```python
from build123d import *

# Parameters (mm, degrees)
BOSS_EXTRUDE1_DEPTH = 15
FILLET1_R           = 2.5


with BuildPart() as part:
    # Sketch1 → Boss-Extrude1 (new body)
    with BuildSketch(Plane.XY):
        with BuildLine():
            Line((4.569752453, 56.5222889), (27.069752453, 56.5222889))
            Line((27.069752453, 56.5222889), (27.069752453, 51.5222889))
            Line((27.069752453, 51.5222889), (4.569751288, 51.5222889))
            ThreePointArc((4.569751288, 51.5222889), (-15.430247547, 31.522287735), (4.569753619, 11.5222889))
            ThreePointArc((4.569753619, 11.5222889), (29.569753619, -13.4777111), (4.569753619, -38.4777111))
            Line((4.569753619, -38.4777111), (-17.930246381, -38.4777111))
            Line((-17.930246381, -38.4777111), (-17.930246381, -33.4777111))
            Line((-17.930246381, -33.4777111), (4.569753619, -33.4777111))
            ThreePointArc((4.569753619, -33.4777111), (24.569753619, -13.477710841), (4.569753101, 6.5222889))
            ThreePointArc((4.569753101, 6.5222889), (-20.430247547, 31.522288577), (4.569752453, 56.5222889))
        make_face()
    extrude(amount=BOSS_EXTRUDE1_DEPTH)

    # Fillet1
    fillet1_edges = [part.edges().sort_by_distance(p)[0] for p in [
        (-17.930246381, -38.4777111, 7.5),
        (-17.930246381, -33.4777111, 7.5),
        (27.069752453, 51.5222889, 7.5),
        (27.069752453, 56.5222889, 7.5),
    ]]
    fillet(fillet1_edges, radius=FILLET1_R - 0.0001)  # a hair under: the kernel refuses the full size


solid = part.part
```
Part model, mm, in its own coordinate system. A direction names the side the tool comes from. Round coordinates to 2 decimals unless told otherwise and drop trailing zeros. Write each loop counter-clockwise with the first axis right and the second up, starting at its lowest first coordinate (ties: lowest second). Pieces come first, ordered by that corner, then holes. Notation, with made-up numbers: (61, 86.5) -> (95, 86.5) arc R11 cw to (95, 95.5) -> close; hole circle Ø10 at (9.25, -2.5). An arc over 180 degrees is marked (long way). Return JSON: item names as keys, results as strings. Group by question number.
Q1. Saw through at A-A on x = 8.5. Write the cut outline in (y, z).
Q2. Saw through at D-D on x = 2. Write the cut outline in (y, z).
Q3. Mould opens along Y. For faces 1 (the flat face through (1, 9, 15)), 2 (the flat face through (14, 56.522, 7)), 3 (the cylindrical face through (-20.424, 30.973, 7.395)) say: pulls with the +Y half, pulls with the -Y half, needs draft (parallel to the pull), parting line crosses it, or undercut.
Q4. Pin check, flat tips, straight feed: pin 1 (3 mm diameter, centred on x = -1.5, z = 11.5, fed in from +Y); pin 2 (2 mm diameter, centred on y = -1.5, z = 5, fed in from -X); pin 3 (4 mm diameter, centred on y = -11.5, z = 4.5, fed in from +X). Stop position of each tip, or through.
Q5. Probe L1, parallel to Y at x = 12.5, z = 2; L2, parallel to Y at x = 11.5, z = 5.25; L3, parallel to X at y = -13, z = 5.75. List the from-to ranges inside material, lowest first. Write a range as [from, to].
Q6. Which spindle directions (+Z, -Z, +X, -X, +Y, -Y) get a long thin tool onto all of the face, cutting with end or side? Do faces 4 (the flat face through (-6, -33.478, 7)), 5 (the cylindrical face through (26.357, 52.274, 7.605)), 6 (the cylindrical face through (26.32, 55.81, 7.6)). Say none if no direction does.
Q7. Saw through at C-C on x = -17. Write the cut outline in (y, z), plus the area to 3 significant figures.
Answer:
{
 "1": {"outline": "(-38.17, 0) -> (-33.09, 0) -> (-33.09, 15) -> (-38.17, 15) -> close; (6.13, 0) -> (11.21, 0) -> (11.21, 15) -> (6.13, 15) -> close; (51.52, 0) -> (56.52, 0) -> (56.52, 15) -> (51.52, 15) -> close"},
 "2": {"outline": "(-38.48, 0) -> (-33.48, 0) -> (-33.48, 15) -> (-38.48, 15) -> close; (6.65, 0) -> (11.69, 0) -> (11.69, 15) -> (6.65, 15) -> close; (51.36, 0) -> (56.39, 0) -> (56.39, 15) -> (51.36, 15) -> close"},
 "3": {"face 1": "needs draft", "face 2": "pulls with the +Y half", "face 3": "undercut"},
 "4": {"pin 1": "y = 56.1", "pin 2": "x = 19.79", "pin 3": "x = 29.57"},
 "5": {"L1": "[-37.19, -31.84], [4.88, 10.23], [51.52, 56.52]", "L2": "[-37.5, -32.24], [5.28, 10.54], [51.52, 56.52]", "L3": "[24.56, 29.57]"},
 "6": {"face 4": "+Z, -Z, -X", "face 5": "+Z, -Z, +X", "face 6": "+Z, -Z, +X, +Y"},
 "7": {"outline": "(-37.92, 0) -> (-34.03, 0) -> (-34.03, 15) -> (-37.92, 15) -> close; (18.88, 0) -> (44.16, 0) -> (44.16, 15) -> (18.88, 15) -> close", "area": "438 mm2"}
}
